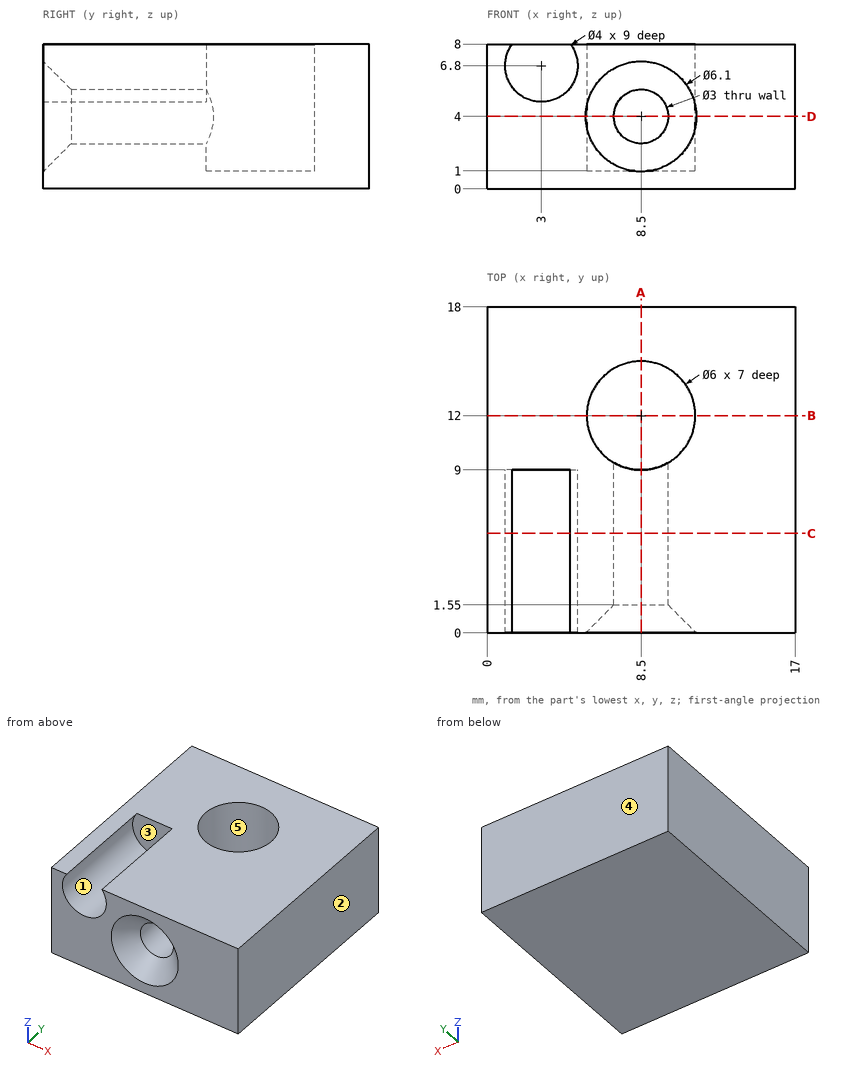
The drawing under review shows one solid part. Ordinate dimensions are in mm from its lowest x, y, z. A direction names the side the tool comes from. Round coordinates to 2 decimals unless told otherwise and drop trailing zeros. Write each loop counter-clockwise with the first axis right and the second up, starting at its lowest first coordinate (ties: lowest second). Pieces come first, ordered by that corner, then holes. Notation, with made-up numbers: (-3, 84.5) - (49, 84.5) arc R36 cw to (49, 123.5) - close; hole circle Ø7 at (-39.5, 10.25). An arc over 180 degrees is marked (long way). Use a Markdown table: item, result. Add a question column.
1. Clearance check with flat-ended pins moving along their axes: pin 1 (3.5 mm diameter, centred on x = 8.5, y = 12, fed in from +Z); pin 2 (2.5 mm diameter, centred on x = 8.5, z = 4, fed in from -Y); pin 3 (1 mm diameter, centred on x = 4, z = 6, fed in from -Y). State where each tip first meets the part, or that it passes through.
2. We need section A-A (x = 8.5). State the section outline as (y, z) points.
3. We need section D-D (z = 4). State the section outline as (x, y) points.
4. For the marked faces 1 and 2, list the 3-axis set-ups (+Z, -Z, +X, -X, +Y, -Y) from which the entire face can be reached by the end or side of a thin tool; tool diameter is ignored.
5. Wall thickness on probe 1 along X at (y, z) = (6.25, 4); probe 2 along X at (y, z) = (5.25, 6.8); probe 3 along Z at (x, y) = (8.5, 7.5): over which ranges is each line inside the solid? List them lowest first.
6. We need section B-B (y = 12). State the section outline as (x, z) points, then the cut area to 3 significant figures.
7. We need section C-C (y = 5.5). State the section outline as (x, z) points.
8. Mouldability with a two-part tool opening along Y and no side actions: class the marked faces 3, 4 and 5 as +Y half, -Y half, draft (parallel to the pull), parting line (faces both ways), or undercut.
Output:
| question | item | result |
|---|---|---|
| 1 | pin 1 | stops at z = 1 |
| 1 | pin 2 | stops at y = 14.73 |
| 1 | pin 3 | stops at y = 9 |
| 2 | outline | (0, 0) - (18, 0) - (18, 8) - (15, 8) - (15, 1) - (9, 1) - (9, 2.5) - (1.55, 2.5) - (0, 0.95) - close; (0, 7.05) - (1.55, 5.5) - (9, 5.5) - (9, 8) - (0, 8) - close |
| 3 | outline | (0, 0) - (5.45, 0) - (7, 1.55) - (7, 9.4) arc R3 cw (long way) to (10, 9.4) - (10, 1.55) - (11.55, 0) - (17, 0) - (17, 18) - (0, 18) - close |
| 4 | face 1 | -Y |
| 4 | face 2 | +Z, -Z, +X, +Y, -Y |
| 5 | probe 1 | x = 0 to 7, 10 to 17 |
| 5 | probe 2 | x = 0 to 1, 5 to 17 |
| 5 | probe 3 | z = 0 to 2.5, 5.5 to 8 |
| 6 | outline | (0, 0) - (17, 0) - (17, 8) - (11.5, 8) - (11.5, 1) - (5.5, 1) - (5.5, 8) - (0, 8) - close |
| 6 | area | 94.0 mm2 |
| 7 | outline | (0, 0) - (17, 0) - (17, 8) - (4.6, 8) arc R2 cw (long way) to (1.4, 8) - (0, 8) - close; hole circle Ø3 at (8.5, 4) |
| 8 | face 3 | -Y half |
| 8 | face 4 | +Y half |
| 8 | face 5 | undercut |
